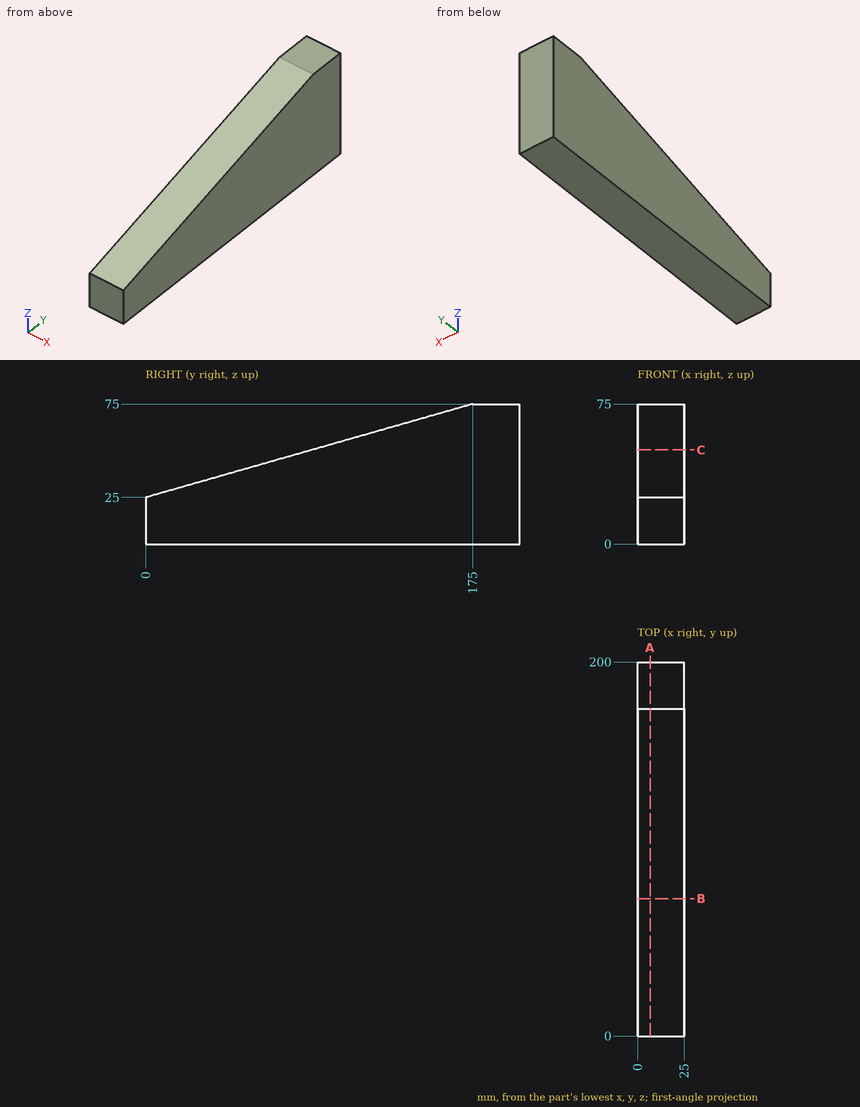
Drawing for the job (mm, zero at the part's lowest x, y, z). Give positions to 0.01 mm unless a question says otherwise; leave off trailing zeros. Order: outer loops, then holes, each group sorted by start corner. A loop starts at its lowest first (then second) coordinate and runs counter-clockwise, first axis right, second up. Notation, with made-up numbers: M -29.75,-15 L 20.25,-15 A17 cw 20.25,9 Z; hole C -1,51.5 d9. An arc over 180 degrees is marked long. Use a Markdown table: item, result. Add a question column.
(1) Probe line 1 along Z through (x, y) = (15.25, 54.5); line 2 along Z through (x, y) = (22.25, 166.5). List the from-to ranges inside material, lowest first. Write a range as [from, to].
(2) Drop a flat-ended pin along its axis: P1, Ø4, axis at x = 20.5, y = 44, coming from the +Z side. Give the stop position or say it passes through.
(3) Saw through at A-A, the plane x = 6.75. Give the cut face in (y, z), and give its area (3 significant figures).
(4) Saw through at B-B, the plane y = 73.5. Give the cut face in (x, z).
(5) Saw through at C-C, the plane z = 50.5. Give the cut face in (x, y), and give its area (3 significant figures).
Answer key:
| question | item | result |
|---|---|---|
| 1 | line 1 | [0, 40.57] |
| 1 | line 2 | [0, 72.57] |
| 2 | P1 | z = 38.14 |
| 3 | outline | M 0,0 L 200,0 L 200,75 L 175,75 L 0,25 Z |
| 3 | area | 10,600 mm^2 |
| 4 | outline | M 0,0 L 25,0 L 25,46 L 0,46 Z |
| 5 | outline | M 0,89.25 L 25,89.25 L 25,200 L 0,200 Z |
| 5 | area | 2,770 mm^2 |
